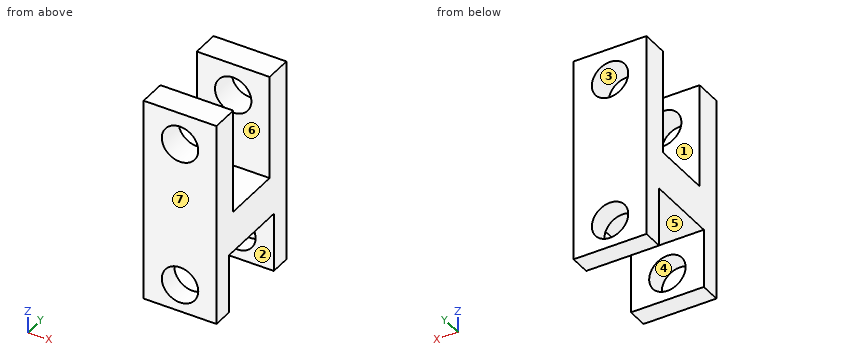
from build123d import *

# Parameters (mm, degrees)
F0_W     = 16
F0_H     = 45
F0_R     = 4
F1_DEPTH = 25
F2_W     = 16
F2_H     = 13
F2_W_2   = 13
F2_H_2   = 23
F3_DEPTH = 16.001


with BuildPart() as f1:
    # F0 (on Front) → F1 (new body)
    with BuildSketch(Plane.XZ):
        with Locations((0, 22.5)):
            Rectangle(F0_W, F0_H)
        with Locations((0, 6)):
            Circle(F0_R, mode=Mode.SUBTRACT)
        with Locations((0, 38)):
            Circle(F0_R, mode=Mode.SUBTRACT)
    extrude(amount=F1_DEPTH)

    # F2 (on face) → F3 (cut, through all)
    with BuildSketch(Plane.YZ.offset(8)):
        with Locations((-12.5, 6.5)):
            Rectangle(F2_W, F2_H)
        with Locations((-12.5, 33.5)):
            Rectangle(F2_W_2, F2_H_2)
    extrude(amount=-F3_DEPTH, mode=Mode.SUBTRACT)


solid = f1.part
Check sheet for the modelled part. Datum: model origin and axes. Units: mm. Face numbers are marked on the shaded views. A direction names the side the tool comes from. Round coordinates to 2 decimals unless told otherwise and drop trailing zeros. Write each loop counter-clockwise with the first axis right and the second up, starting at its lowest first coordinate (ties: lowest second). Pieces come first, ordered by that corner, then holes. Notation, with made-up numbers: (17, 65.5) - (24, 65.5) arc R20 ccw to (24, 72.5) - close; hole circle Ø5 at (82.25, 75). An arc over 180 degrees is marked (long way). Return JSON: item names as keys, results as strings.
Q1. Access from +Z, -Z, +X, -X, +Y, -Y to the whole of each face (thin tool, end or side, straight path). Record for the marked faces 1, 2 and 3.
Returned:
{"face 1": "+Z, +X, -X", "face 2": "-Z, +X, -X", "face 3": "+Y, -Y"}
Q2. Cross-section at B-B (x = 0). Record the boundary of the cut face in (y, z).
Returned:
{"outline": "(-25, 0) - (-20.5, 0) - (-20.5, 2) - (-25, 2) - close; (-25, 10) - (-20.5, 10) - (-20.5, 13) - (-4.5, 13) - (-4.5, 10) - (0, 10) - (0, 34) - (-6, 34) - (-6, 22) - (-19, 22) - (-19, 34) - (-25, 34) - close; (-25, 42) - (-19, 42) - (-19, 45) - (-25, 45) - close; (-6, 42) - (0, 42) - (0, 45) - (-6, 45) - close; (-4.5, 0) - (0, 0) - (0, 2) - (-4.5, 2) - close"}
Q3. Cross-section at C-C (z = 31.5). Record the boundary of the cut face in (x, y).
Returned:
{"outline": "(-8, -25) - (8, -25) - (8, -19) - (-8, -19) - close; (-8, -6) - (8, -6) - (8, 0) - (-8, 0) - close"}
Q4. Cross-section at A-A (z = 6). Record the boundary of the cut face in (x, y).
Returned:
{"outline": "(-8, -25) - (-4, -25) - (-4, -20.5) - (-8, -20.5) - close; (-8, -4.5) - (-4, -4.5) - (-4, 0) - (-8, 0) - close; (4, -25) - (8, -25) - (8, -20.5) - (4, -20.5) - close; (4, -4.5) - (8, -4.5) - (8, 0) - (4, 0) - close"}
Q5. Depth check by flat-ended pin: P1, Ø9, axis at x = 0, z = 6, coming from the -Y side; P2, Ø5, axis at x = -2.5, y = -16, coming from the -Z side; P3, Ø6.5, axis at x = 0, z = 38, coming from the -Y side. Enter the tip coordinate at first touch or a pass-through.
Returned:
{"P1": "stops at y = -25", "P2": "stops at z = 13", "P3": "passes through"}
Q6. Cross-section at D-D (y = -21). Record the boundary of the cut face in (x, z), then the cut area to 3 significant figures.
Returned:
{"outline": "(-8, 0) - (8, 0) - (8, 45) - (-8, 45) - close; hole circle Ø8 at (0, 6); hole circle Ø8 at (0, 38)", "area": "619 mm²"}
Q7. Draft check along Y on the marked faces 4, 5, 6 and 7. Enter one of: released by +Y, released by -Y, zero draft, split by the parting line, or undercut.
Returned:
{"face 4": "zero draft", "face 5": "undercut", "face 6": "undercut", "face 7": "released by -Y"}
Q8. Scan lines: L1, parallel to Z at x = 0, y = -1.3; L2, parallel to Y at x = -3.5, z = 9; L3, parallel to Y at x = -3.5, z = 31. Record each from-to range of solid material in increasing order. Write a range as from..to.
Returned:
{"L1": "z = 0..2, 10..34, 42..45", "L2": "y = -25..-20.5, -4.5..0", "L3": "y = -25..-19, -6..0"}
